The figure shows three views and two pictorial views of one solid part (mm, origin at its lowest corner). Answer the questions. A direction names the side the tool comes from. Coordinates: 2 decimals unless noted, no trailing zeros. Loops run counter-clockwise (first coordinate to the right, second up) from the corner with the lowest first, then second, coordinate; pieces in that order, holes last. Notation, with made-up numbers: M 6.5,29 L 51.5,29 A24 cw 51.5,51 Z; hole C 42.5,54 d11. An arc over 180 degrees is marked long. Return JSON: item names as keys, results as strings. Group by question number.
1. Section C-C (y = 10.75) is taken. Write down the section's boundary in (x, z), then the cut area to 3 significant figures.
2. Given P1, Ø6, axis at x = 9, y = 7.5, coming from the +Z side; P2, Ø2, axis at x = 7.5, y = 24, coming from the +Z side; P3, Ø2, axis at x = 3, z = 17, coming from the +Y side, each flat-ended and moving along its own axis, determine where each tip first touches the part or whether it passes through.
3. Straight lines are drawn through the part: L1, parallel to Y at x = 1.75, z = 18.5; L2, parallel to Y at x = 11, z = 13; L3, parallel to X at y = 24.75, z = 19.5 (1 decimal). For each, find the intervals that lie inside material, in ascending order. Write a range as from..to.
4. Section D-D (x = 3) is taken. Write down the section's boundary in (y, z).
5. Which of the six approach directions +Z, -Z, +X, -X, +Y, -Y give full straight-line access (tool end or side, diameter ignored) to the marked faces 1, 2, 3 and 4?
6. Section A-A (x = 6) is taken. Write down the section's boundary in (y, z), then the cut area to 3 significant figures.
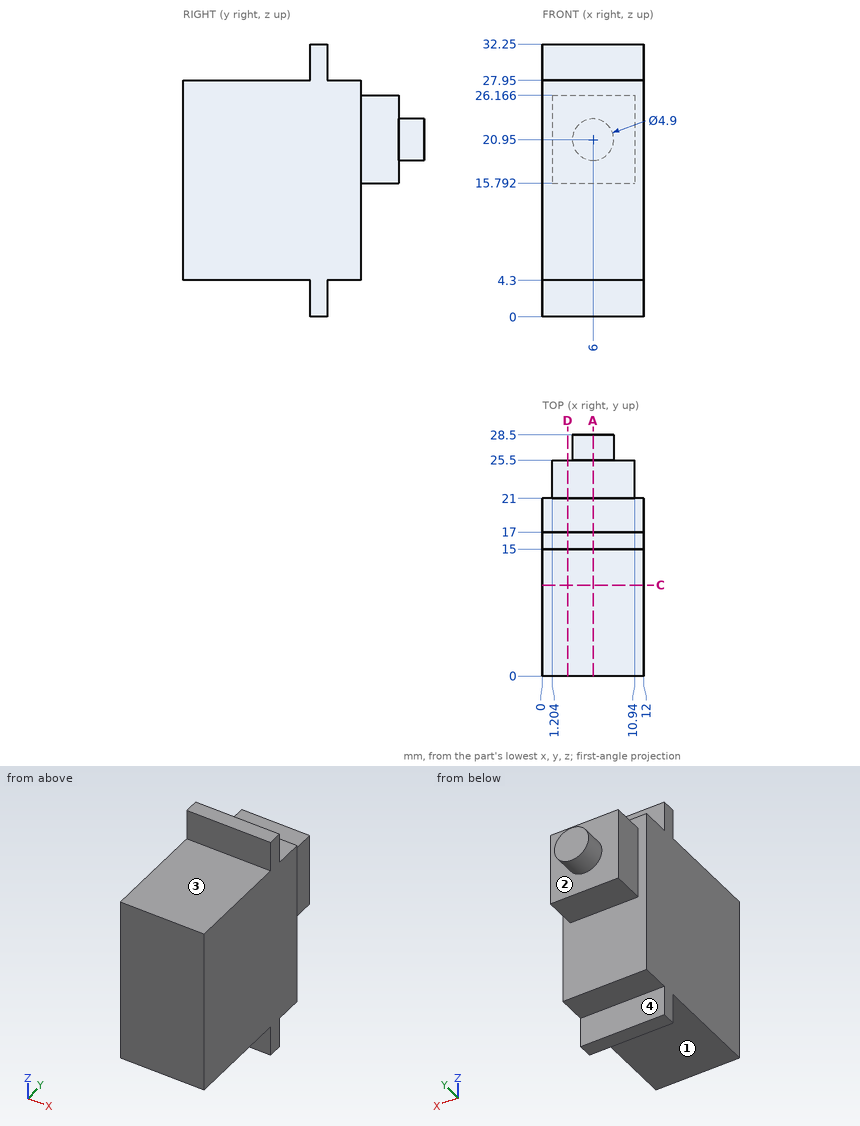
Worked out:
{
 "1": {"outline": "M 0,4.3 L 12,4.3 L 12,27.95 L 0,27.95 Z", "area": "284 mm^2"},
 "2": {"P1": "z = 27.95", "P2": "z = 26.17", "P3": "y = 25.5"},
 "3": {"L1": "0..25.5", "L2": "0..21", "L3": "1.2..10.9"},
 "4": {"outline": "M 0,4.3 L 15,4.3 L 15,0 L 17,0 L 17,4.3 L 21,4.3 L 21,15.79 L 25.5,15.79 L 25.5,26.17 L 21,26.17 L 21,27.95 L 17,27.95 L 17,32.25 L 15,32.25 L 15,27.95 L 0,27.95 Z"},
 "5": {"face 1": "-Z, +X, -X, -Y", "face 2": "+Y", "face 3": "+Z, +X, -X, -Y", "face 4": "-Z, +X, -X, +Y"},
 "6": {"outline": "M 0,4.3 L 15,4.3 L 15,0 L 17,0 L 17,4.3 L 21,4.3 L 21,15.79 L 25.5,15.79 L 25.5,18.5 L 28.5,18.5 L 28.5,23.4 L 25.5,23.4 L 25.5,26.17 L 21,26.17 L 21,27.95 L 17,27.95 L 17,32.25 L 15,32.25 L 15,27.95 L 0,27.95 Z", "area": "575 mm^2"}
}
